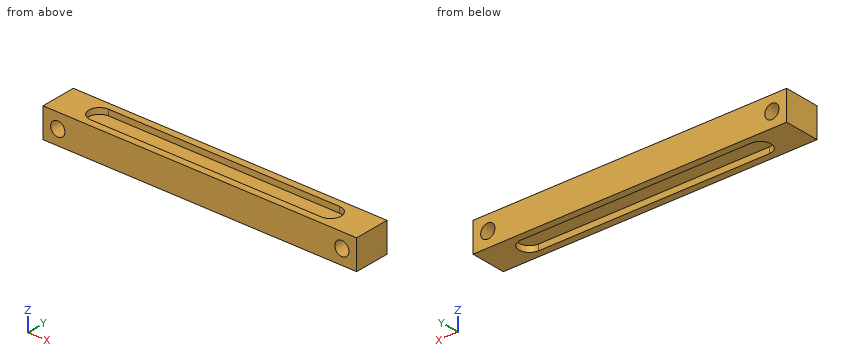
from build123d import *

# Parameters (mm, degrees)
SKETCH1_W           = 336.55
SKETCH1_H           = 31.75
SKETCH1_R           = 7.62
BOSS_EXTRUDE1_DEPTH = 38.1
CUT_EXTRUDE1_DEPTH  = 6.35
CUT_EXTRUDE3_START  = -6.35
CUT_EXTRUDE3_DEPTH  = 6.35


with BuildPart() as part:
    # Sketch1 → Boss-Extrude1 (new body)
    with BuildSketch(Plane(origin=(0, 0, 0), x_dir=(1, 0, 0), z_dir=(0, 1, 0))):
        with Locations((168.275, 15.875)):
            Rectangle(SKETCH1_W, SKETCH1_H)
        with Locations(Location((15.875, 15.875, 0), (0, 0, 90))):
            Circle(SKETCH1_R, mode=Mode.SUBTRACT)
        with Locations(Location((320.675, 15.875, 0), (0, 0, 90))):
            Circle(SKETCH1_R, mode=Mode.SUBTRACT)
    extrude(amount=BOSS_EXTRUDE1_DEPTH)

    # Sketch4 → Cut-Extrude1 (cut)
    with BuildSketch(Plane.XY):
        with BuildLine():
            Line((44.45, 30.48), (292.1, 30.48))
            ThreePointArc((292.1, 30.48), (303.53, 19.05), (292.1, 7.62))
            Line((292.1, 7.62), (44.45, 7.62))
            ThreePointArc((44.45, 7.62), (33.02, 19.05), (44.45, 30.48))
        make_face()
    extrude(amount=-CUT_EXTRUDE1_DEPTH, mode=Mode.SUBTRACT)

    # Sketch6 → Cut-Extrude3 (cut)
    with BuildSketch(Plane(origin=(0, 0, -31.75), x_dir=(-1, 0, 0), z_dir=(0, 0, -1)).offset(CUT_EXTRUDE3_START)):
        with BuildLine():
            Line((-292.1, 30.48), (-44.45, 30.48))
            ThreePointArc((-44.45, 30.48), (-33.02, 19.05), (-44.45, 7.62))
            Line((-44.45, 7.62), (-292.1, 7.62))
            ThreePointArc((-292.1, 7.62), (-303.53, 19.05), (-292.1, 30.48))
        make_face()
    extrude(amount=CUT_EXTRUDE3_DEPTH, mode=Mode.SUBTRACT)


solid = part.part
Here's how the part is built. I have some questions about the finished solid (model axes, mm). Coordinates: 2 decimals unless noted, no trailing zeros. Order: outer loops, then holes, each group sorted by start corner. A loop starts at its lowest first (then second) coordinate and runs counter-clockwise, first axis right, second up. Notation, with made-up numbers: (-28, 47) -> (1, 47) arc R18 ccw to (1, 80) -> close; hole circle Ø3 at (41.5, -21.5). An arc over 180 degrees is marked (long way). Answer in a Markdown table with one row per item.
(1) Please list where these lines run through material, in increasing order: probe 1 along Y at (x, z) = (229.5, -3); probe 2 along X at (y, z) = (16, -19.5); probe 3 along X at (y, z) = (6.5, -9).
Answer key:
| item | result |
|---|---|
| probe 1 | 0 to 7.62, 30.48 to 38.1 |
| probe 2 | 0 to 9.17, 22.58 to 313.97, 327.38 to 336.55 |
| probe 3 | 0 to 12.59, 19.16 to 317.39, 323.96 to 336.55 |
(2) I want a section at C-C on y = 15.5. List the corners of the cut face in (x, z) for me (3 decimals).
Answer key:
| item | result |
|---|---|
| outline | (0, -31.75) -> (33.585, -31.75) -> (33.585, -25.4) -> (302.965, -25.4) -> (302.965, -31.75) -> (336.55, -31.75) -> (336.55, 0) -> (302.965, 0) -> (302.965, -6.35) -> (33.585, -6.35) -> (33.585, 0) -> (0, 0) -> close; hole circle Ø15.24 at (15.875, -15.875); hole circle Ø15.24 at (320.675, -15.875) |
(3) Will these pins go through, and if not, where does the flat tip stop? pin 1 Ø2 at (x, y) = (194.5, 27) entering from -Z; pin 2 Ø13.5 at (x, z) = (15.875, -15.875) entering from +Y; pin 3 Ø11.5 at (x, y) = (143.5, 18.5) entering from +Z.
Answer key:
| item | result |
|---|---|
| pin 1 | z = -25.4 |
| pin 2 | through |
| pin 3 | z = -6.35 |
(4) I want a section at B-B on z = -16. List the corners of the cut face in (x, y) for me.
Answer key:
| item | result |
|---|---|
| outline | (0, 0) -> (8.26, 0) -> (8.26, 38.1) -> (0, 38.1) -> close; (23.49, 0) -> (313.06, 0) -> (313.06, 38.1) -> (23.49, 38.1) -> close; (328.29, 0) -> (336.55, 0) -> (336.55, 38.1) -> (328.29, 38.1) -> close |
(5) I want a section at A-A on x = 217.5. List the corners of the cut face in (y, z) for me, then the cut area to 3 significant figures.
Answer key:
| item | result |
|---|---|
| outline | (0, -31.75) -> (7.62, -31.75) -> (7.62, -25.4) -> (30.48, -25.4) -> (30.48, -31.75) -> (38.1, -31.75) -> (38.1, 0) -> (30.48, 0) -> (30.48, -6.35) -> (7.62, -6.35) -> (7.62, 0) -> (0, 0) -> close |
| area | 919 mm^2 |
(6) I want a section at D-D on y = 34. List the corners of the cut face in (x, z) for me (3 decimals), then the cut area to 3 significant figures.
Answer key:
| item | result |
|---|---|
| outline | (0, -31.75) -> (336.55, -31.75) -> (336.55, 0) -> (0, 0) -> close; hole circle Ø15.24 at (15.875, -15.875); hole circle Ø15.24 at (320.675, -15.875) |
| area | 10,300 mm^2 |
